```python
from build123d import *

# Parameters (mm, degrees)
SKETCH1_R           = 3.2639
BOSS_EXTRUDE1_DEPTH = 3.175
FILLET1_R           = 4.7625
SKETCH2_R           = 3.2639
CUT_EXTRUDE1_DEPTH  = 3.175


with BuildPart() as part:
    # Sketch1 → Boss-Extrude1 (new body)
    with BuildSketch(Plane.XY):
        Polygon((200.996661906, 21.487802882), (190.846331975, 21.044629906), (191.954264414, -4.331194922), (202.104594345, -3.888021946), align=None)
        with Locations((196.85, 0)):
            Circle(SKETCH1_R, mode=Mode.SUBTRACT)
        with Locations((196.100926319, 17.15660796)):
            Circle(SKETCH1_R, mode=Mode.SUBTRACT)
    extrude(amount=BOSS_EXTRUDE1_DEPTH)

    # Fillet1
    fillet1_edges = [part.edges().sort_by_distance(p)[0] for p in [
        (202.104594345, -3.888021946, 1.5875),
        (191.954264414, -4.331194922, 1.5875),
        (190.846331975, 21.044629906, 1.5875),
        (200.996661906, 21.487802882, 1.5875),
    ]]
    fillet(fillet1_edges, radius=FILLET1_R)

    # Sketch2 → Cut-Extrude1 (cut)
    with BuildSketch(Plane(origin=(191.400298194, 8.356717492, 0), x_dir=(0, 0, 1), z_dir=(-0.9990482215818578, -0.043619387365334696, 0))):
        with Locations((3.96875, 0)):
            Circle(SKETCH2_R)
    extrude(amount=-CUT_EXTRUDE1_DEPTH, mode=Mode.SUBTRACT)


solid = part.part
```
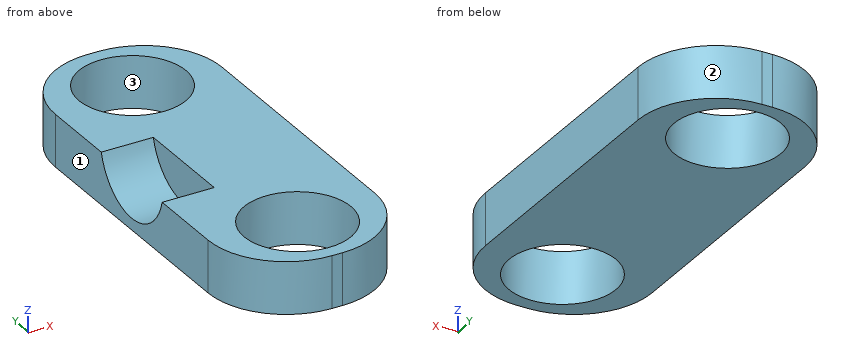
Here's how the part is built. I have some questions about the finished solid (model axes, mm). Face numbers are marked on the shaded views. Give positions to 0.01 mm unless a question says otherwise; leave off trailing zeros. Write each loop counter-clockwise with the first axis right and the second up, starting at its lowest first coordinate (ties: lowest second). Pieces come first, ordered by that corner, then holes.
(1) Thinking about a two-plate mould opening in Y: for the marked faces 1, 2 and 3, which applies, pulls with the +Y half, pulls with the -Y half, needs draft (parallel to the pull), parting line crosses it, or undercut?
Output values:
face 1: pulls with the -Y half
face 2: pulls with the +Y half
face 3: undercut
(2) If I drill on L1, parallel to Y at x = 194, z = 2.05; L2, parallel to Y at x = 195, z = 1.75; L3, parallel to Y at x = 197.25, z = 2.4, over which ranges is the centre line in solid material (lowest first)?
Output values:
L1: y = -3.42 to -1.59, 1.59 to 5.83, 11.11 to 14.66, 19.65 to 20.9
L2: y = -3.88 to -2.69, 2.69 to 14.08, 20.23 to 21.19
L3: y = -4.1 to -3.24, 3.24 to 14.1, 20.21 to 21.22
(3) Imagine slicing it at D-D, the plane y = -1.25. Write out the boundary of the cut face in (x, z) (3 decimals), and give its area (3 significant figures).
Output values:
outline: (192.131, 0) - (193.835, 0) - (193.835, 3.175) - (192.131, 3.175) - close; (199.865, 0) - (201.501, 0) - (201.501, 3.175) - (199.865, 3.175) - close
area: 10.6 mm2
(4) Imagine slicing it at A-A, the plane x = 198. Write out the boundary of the cut face in (y, z) (3 decimals).
Output values:
outline: (-4.022, 0) - (-3.055, 0) - (-3.055, 3.175) - (-4.022, 3.175) - close; (3.055, 0) - (14.502, 0) - (14.502, 3.175) - (3.055, 3.175) - close; (19.811, 0) - (21.024, 0) - (21.024, 3.175) - (19.811, 3.175) - close
(5) Imagine slicing it at C-C, the plane y = 18.5. Write out the boundary of the cut face in (x, z) (3 decimals), and give its area (3 significant figures).
Output values:
outline: (191.492, 0) - (193.126, 0) - (193.126, 3.175) - (191.492, 3.175) - close; (199.076, 0) - (200.779, 0) - (200.779, 3.175) - (199.076, 3.175) - close
area: 10.6 mm2
(6) Imagine slicing it at B-B, the plane z = 2.45. Count the separate pieces of the cut face and the enclosed holes in it, and give its area (3 significant figures).
Output values:
separate pieces: 1
enclosed holes: 2
area: 153 mm2
